Autodesk Inventor part; units mm, degrees
ref_plane "YZ Plane" through (0, 0, 0) normal (1, 0, 0) x (0, 1, 0)
ref_plane "XZ Plane" through (0, 0, 0) normal (0, 1, 0) x (-1, 0, 0)
ref_plane "XY Plane" through (0, 0, 0) normal (0, 0, 1) x (1, 0, 0)
sketch "Sketch1" plane through (0, 0, 0) normal (0, 0, 1) x (1, 0, 0)
  line L0 (-12.7, 25.4) -> (12.7, 25.4)
  line L1 (12.7, 25.4) -> (12.7, -25.4)
  line L2 (12.7, -25.4) -> (-12.7, -25.4)
  line L3 (-12.7, -25.4) -> (-12.7, 25.4)
  line L4 (9.525, 22.225) -> (-9.525, 22.225)
  line L5 (-9.525, 22.225) -> (-9.525, -22.225)
  line L6 (-9.525, -22.225) -> (9.525, -22.225)
  line L7 (9.525, -22.225) -> (9.525, 22.225)
  point P0 (0, 0)
  point P1 (0, 25.4)
  point P2 (-12.7, 0)
extrude "Extrusion1" add sketch "Sketch1" along normal mid plane 304.8
properties part number "Aluminum Box Tube" material "Aluminum 6061"
The model under review builds one solid part; all positions refer to its coordinate system, in mm. A direction names the side the tool comes from. Coordinates: 2 decimals unless noted, no trailing zeros. Write each loop counter-clockwise with the first axis right and the second up, starting at its lowest first coordinate (ties: lowest second). Pieces come first, ordered by that corner, then holes. Notation, with made-up numbers: (-0.75, -14.5) - (52.25, -14.5) arc R13 ccw to (52.25, -5.5) - close; hole circle Ø11 at (54.5, 15.5). An arc over 180 degrees is marked (long way). Answer in a Markdown table with one row per item. Add a question column.
Q1. Consider section C-C on x = 3.5. Give the boundary of the cut face in (y, z) (3 decimals), then the cut area to 3 significant figures.
Q2. Consider section A-A on y = -16. Give the boundary of the cut face in (x, z) (3 decimals).
Q3. Consider section B-B on z = 115. Give the boundary of the cut face in (x, y) (3 decimals), then the cut area to 3 significant figures.
Q4. For faces 4 (the face through (0, -22.225, -2)), 5 (the face through (0, -25.4, -2)), list the 3-axis set-ups (+Z, -Z, +X, -X, +Y, -Y) from which the entire face can be reached by the end or side of a thin tool; tool diameter is ignored.
Q5. Draft analysis for pull direction X (two halves, no side actions). For faces 1 (the face through (0, 22.225, -2)), 2 (the face through (-10, -2, 152.4)), 3 (the face through (-12.7, 0, -2)), state which applies: +X half, -X half, draft (parallel to the pull), parting line (faces both ways), or undercut.
Q6. To check wall thickness, follow line 1 along X through (y, z) = (-5.5, 101.5) (3 decimals); line 2 along Y through (x, z) = (-0.75, -53) (3 decimals). State the ranges of each line that lie inside material, in increasing order. Write a range as from..to.
Answers below:
| question | item | result |
|---|---|---|
| 1 | outline | (-25.4, -152.4) - (-22.225, -152.4) - (-22.225, 152.4) - (-25.4, 152.4) - close; (22.225, -152.4) - (25.4, -152.4) - (25.4, 152.4) - (22.225, 152.4) - close |
| 1 | area | 1,940 mm² |
| 2 | outline | (-12.7, -152.4) - (-9.525, -152.4) - (-9.525, 152.4) - (-12.7, 152.4) - close; (9.525, -152.4) - (12.7, -152.4) - (12.7, 152.4) - (9.525, 152.4) - close |
| 3 | outline | (-12.7, -25.4) - (12.7, -25.4) - (12.7, 25.4) - (-12.7, 25.4) - close; hole (-9.525, -22.225) - (9.525, -22.225) - (9.525, 22.225) - (-9.525, 22.225) - close |
| 3 | area | 444 mm² |
| 4 | face 4 | +Z, -Z |
| 4 | face 5 | +Z, -Z, +X, -X, -Y |
| 5 | face 1 | undercut |
| 5 | face 2 | draft |
| 5 | face 3 | -X half |
| 6 | line 1 | -12.7..-9.525, 9.525..12.7 |
| 6 | line 2 | -25.4..-22.225, 22.225..25.4 |
